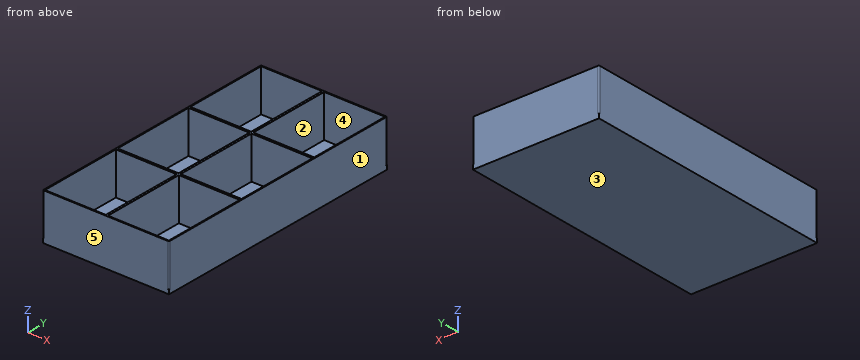
from build123d import *

# Parameters (mm, degrees)
F0_W     = 29
F0_H     = 40
F1_DEPTH = 20
F2_R     = 0.5
F3_W     = 60
F3_H     = 123
F4_DEPTH = 2


with BuildPart() as f1:
    # F0 (on Top) → F1 (new body)
    with BuildSketch(Plane.XY):
        Polygon((-15, 61.5), (-30, 61.5), (-30, 20.5), (-30, -20.5), (-30, -61.5), (0, -61.5), (15, -61.5), (30, -61.5), (30, 61.5), (15, 61.5), (0, 61.5), align=None)
        with Locations((-15, -41)):
            Rectangle(F0_W, F0_H, mode=Mode.SUBTRACT)
        Polygon((0.5, -21), (15, -21), (29.5, -21), (29.5, -61), (0.5, -61), align=None, mode=Mode.SUBTRACT)
        with Locations((-15, 0)):
            Rectangle(F0_W, F0_H, mode=Mode.SUBTRACT)
        Polygon((-29.5, 61), (-15, 61), (-0.5, 61), (-0.5, 21), (-29.5, 21), align=None, mode=Mode.SUBTRACT)
        Polygon((0.5, -20), (0.5, 20), (29.5, 20), (29.5, -20), (15, -20), align=None, mode=Mode.SUBTRACT)
        Polygon((0.5, 61), (15, 61), (29.5, 61), (29.5, 21), (0.5, 21), align=None, mode=Mode.SUBTRACT)
    extrude(amount=F1_DEPTH)

    # F2
    f2_edges = [f1.edges().sort_by_distance(p)[0] for p in [
        (30, 61.5, 10),
        (30, -61.5, 10),
        (-30, -61.5, 10),
        (-30, 61.5, 10),
    ]]
    fillet(f2_edges, radius=F2_R)

    # F3 (on Top) → F4 (join)
    with BuildSketch(Plane.XY):
        Rectangle(F3_W, F3_H)
    extrude(amount=-F4_DEPTH)


solid = f1.part
Geometry check sheet. Reference: the model listing, model coordinates, mm. Face numbers are marked on the shaded views. A direction names the side the tool comes from. Coordinates: 2 decimals unless noted, no trailing zeros. Order: outer loops, then holes, each group sorted by start corner. A loop starts at its lowest first (then second) coordinate and runs counter-clockwise, first axis right, second up. Notation, with made-up numbers: (33.5, 62) -> (57.5, 62) arc R21 ccw to (57.5, 92) -> close; hole circle Ø6 at (51, -4). An arc over 180 degrees is marked (long way). Use a Markdown table: item, result. Add a question column.
1. Mould release check, pull along X, two halves, no side actions. Record for the marked faces 1, 2 and 3: pulls with the +X half, pulls with the -X half, needs draft (parallel to the pull), parting line crosses it, or undercut.
2. Set-up check for the marked faces 4 and 5: record each of +Z, -Z, +X, -X, +Y, -Y from which the full face is reachable in a straight line by a thin tool's end or side.
3. Cross-section at A-A (z = 5.75). Give the number of separate pieces and of enclosed holes in the cut face, and give its area (3 significant figures).
4. Material ranges on L1, parallel to X at y = 25.5, z = 5.5; L2, parallel to Y at x = -3.5, z = 12.25; L3, parallel to Z at x = 9, y = -15.5, recorded low to high.
5. Go/stop test with a flat-tipped pin: pin 1 Ø1 at (x, y) = (10, -37.5) entering from +Z. Record where the tip stops, or that it passes through.
6. Cross-section at C-C (y = 13). Enter the section's corners in (x, z), and give its area (3 significant figures).
7. Cross-section at B-B (x = -23). Enter the section's corners in (y, z), and give its area (3 significant figures).
Filled sheet:
| question | item | result |
|---|---|---|
| 1 | face 1 | pulls with the +X half |
| 1 | face 2 | undercut |
| 1 | face 3 | needs draft |
| 2 | face 4 | +Z |
| 2 | face 5 | +Z, -Z, +X, -X, -Y |
| 3 | separate pieces | 1 |
| 3 | enclosed holes | 6 |
| 3 | area | 420 mm2 |
| 4 | L1 | -30 to -29.5, -0.5 to 0.5, 29.5 to 30 |
| 4 | L2 | -61.5 to -61, -21 to -20, 20 to 21, 61 to 61.5 |
| 4 | L3 | -2 to 0 |
| 5 | pin 1 | z = 0 |
| 6 | outline | (-30, -2) -> (30, -2) -> (30, 20) -> (29.5, 20) -> (29.5, 0) -> (0.5, 0) -> (0.5, 20) -> (-0.5, 20) -> (-0.5, 0) -> (-29.5, 0) -> (-29.5, 20) -> (-30, 20) -> close |
| 6 | area | 160 mm2 |
| 7 | outline | (-61.5, -2) -> (61.5, -2) -> (61.5, 20) -> (61, 20) -> (61, 0) -> (21, 0) -> (21, 20) -> (20, 20) -> (20, 0) -> (-20, 0) -> (-20, 20) -> (-21, 20) -> (-21, 0) -> (-61, 0) -> (-61, 20) -> (-61.5, 20) -> close |
| 7 | area | 306 mm2 |
